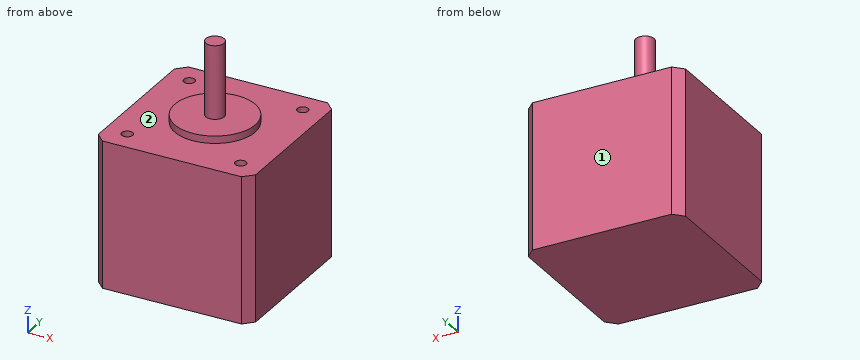
```python
from build123d import *

# Parameters (mm, degrees)
SKETCH1_W           = 43
SKETCH1_H           = 43
BOSS_EXTRUDE1_DEPTH = 40
CHAMFER1_SIZE       = 2.5
SKETCH2_R           = 11
BOSS_EXTRUDE2_DEPTH = 2
SKETCH3_R           = 2.5
BOSS_EXTRUDE3_DEPTH = 20
SKETCH4_R           = 1.5
CUT_EXTRUDE1_DEPTH  = 10


with BuildPart() as part:
    # Sketch1 → Boss-Extrude1 (new body)
    with BuildSketch(Plane.XY):
        Rectangle(SKETCH1_W, SKETCH1_H)
    extrude(amount=BOSS_EXTRUDE1_DEPTH)

    # Chamfer1
    chamfer1_edges = [part.edges().sort_by_distance(p)[0] for p in [
        (21.5, -21.5, 20),
        (-21.5, -21.5, 20),
        (-21.5, 21.5, 20),
        (21.5, 21.5, 20),
    ]]
    chamfer(chamfer1_edges, length=CHAMFER1_SIZE)

    # Sketch2 → Boss-Extrude2 (add)
    with BuildSketch(Plane.XY.offset(40)):
        Circle(SKETCH2_R)
    extrude(amount=BOSS_EXTRUDE2_DEPTH)

    # Sketch3 → Boss-Extrude3 (add)
    with BuildSketch(Plane.XY.offset(42)):
        Circle(SKETCH3_R)
    extrude(amount=BOSS_EXTRUDE3_DEPTH)

    # Sketch4 → Cut-Extrude1 (cut)
    with BuildSketch(Plane.XY.offset(40)):
        with Locations((-15.5, 15.5)):
            Circle(SKETCH4_R)
        with Locations((15.5, 15.5)):
            Circle(SKETCH4_R)
        with Locations((15.5, -15.5)):
            Circle(SKETCH4_R)
        with Locations((-15.5, -15.5)):
            Circle(SKETCH4_R)
    extrude(amount=-CUT_EXTRUDE1_DEPTH, mode=Mode.SUBTRACT)


solid = part.part
```
Design review of the part built by this model. Coordinates are the model's own, in mm. Face numbers are marked on the shaded views. A direction names the side the tool comes from. Coordinates: 2 decimals unless noted, no trailing zeros. Write each loop counter-clockwise with the first axis right and the second up, starting at its lowest first coordinate (ties: lowest second). Pieces come first, ordered by that corner, then holes.
1) Add section A-A (y = -15.5). Write out the cut boundary in (x, z).
2) Add section C-C (z = 50.5). Write out the cut boundary in (x, y), plus the area to 3 significant figures.
3) Add section D-D (x = -9.5). Write out the cut boundary in (y, z).
4) To check wall thickness, follow L1, parallel to Y at x = 15.5, z = 33.25; L2, parallel to Y at x = -15, z = 37; L3, parallel to Z at x = -7, y = 2. State the ranges of each line that lie inside material, in increasing order.
5) Insertion check: pin 1 (4 mm diameter, centred on x = 10.5, y = 4, fed in from +Z); pin 2 (1.5 mm diameter, centred on x = -15.5, y = 16, fed in from +Z); pin 3 (2.5 mm diameter, centred on x = 15.5, y = 16, fed in from +Z). Each pin has a flat end and moves straight along its axis. Give the tip position at first contact, or say it passes through.
6) Machinability: for the marked faces 1 and 2, which of the approach directions +Z, -Z, +X, -X, +Y, -Y give a long, thin tool a straight path to every point of the face, cutting with its end or side? Answer none if there is none.
Check result:
1. outline: (-21.5, 0) - (21.5, 0) - (21.5, 40) - (17, 40) - (17, 30) - (14, 30) - (14, 40) - (-14, 40) - (-14, 30) - (-17, 30) - (-17, 40) - (-21.5, 40) - close
2. outline: circle Ø5 at (0, 0)
2. area: 19.6 mm2
3. outline: (-21.5, 0) - (21.5, 0) - (21.5, 40) - (5.55, 40) - (5.55, 42) - (-5.55, 42) - (-5.55, 40) - (-21.5, 40) - close
4. L1: y = -21.5 to -17, -14 to 14, 17 to 21.5
4. L2: y = -21.5 to -16.91, -14.09 to 14.09, 16.91 to 21.5
4. L3: z = 0 to 42
5. pin 1: stops at z = 42
5. pin 2: stops at z = 30
5. pin 3: stops at z = 40
6. face 1: +Z, -Z, +X, -X, +Y
6. face 2: +Z
